Here's how the part is built. I have some questions about the finished solid (model axes, mm). Round coordinates to 2 decimals unless told otherwise and drop trailing zeros. Loops run counter-clockwise (first coordinate to the right, second up) from the corner with the lowest first, then second, coordinate; pieces in that order, holes last. Notation, with made-up numbers: (86.25, 73.5) - (101.25, 73.5) arc R17 cw to (101.25, 97.5) - close; hole circle Ø3 at (82, 83.25). An arc over 180 degrees is marked (long way). Answer as a JSON object with one key per item and string values. Group by question number.
1) I want a section at C-C, the plane y = -53.5. Please give me the cut outline in (x, z), then the cut area to 3 significant figures.
2) I want a section at A-A, the plane z = 255. Please give me the cut outline in (x, y).
3) I want a section at D-D, the plane z = 167. Please give me the cut outline in (x, y), then the cut area to 3 significant figures.
4) I want a section at B-B, the plane x = 0.1. Please give me the cut outline in (y, z).
5) Will these pins go through, and if not, where does the flat tip stop? P1, Ø1.5, axis at x = -1, z = 190.5, coming from the -Y side (3 decimals); P2, Ø0.9, axis at x = 0, z = 214.5, coming from the -Y side (3 decimals); P3, Ø0.9, axis at x = -0.5, y = 0, coming from the +Z side.
6) If I drill on line 1 along Y through (x, z) = (-1, 279.5); line 2 along Y through (x, z) = (0.5, 181); line 3 along Z through (x, y) = (0.15, -130), over which ranges is the centre line in solid material (lowest first)? Write a range as [from, to].
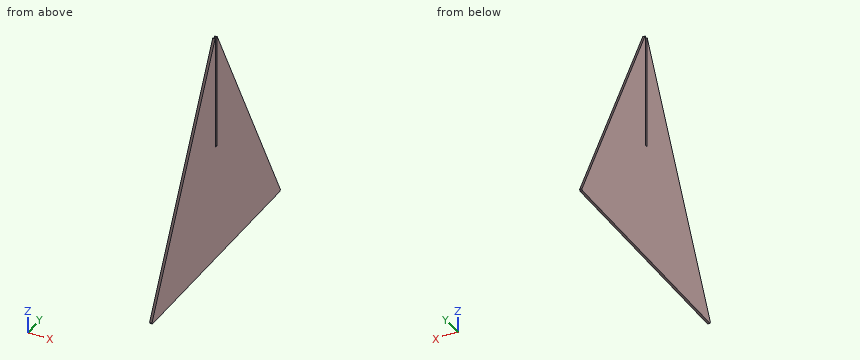
Autodesk Inventor part; units mm, degrees
ref_plane "YZ Plane" through (0, 0, 0) normal (1, 0, 0) x (0, 1, 0)
ref_plane "XZ Plane" through (0, 0, 0) normal (0, 1, 0) x (-1, 0, 0)
ref_plane "XY Plane" through (0, 0, 0) normal (0, 0, 1) x (1, 0, 0)
sketch "Sketch1" plane through (0, 0, 0) normal (1, 0, 0) x (0, 1, 0)
  line L0 (150, 0) -> (-150, 0)
  line L1 (0, 0) -> (0, 300)
  line L2 (0, 300) -> (150, 0)
  line L3 (0, 300) -> (-150, 0)
  dimension "d0" = 300
  dimension "d1" = 300
extrude "Plate1" add sketch "Sketch1" along normal mid plane 3
sketch "Sketch2" plane through (-1.5, 0, 0) normal (-1, 0, 0) x (0, 0, 1)
  line L0 (300, -1.6) -> (149, -1.6)
  line L1 (149, -1.6) -> (149, 1.6)
  line L2 (149, 1.6) -> (300, 1.6)
  line L3 (300, 1.6) -> (300, -1.6)
  point P0 (0, 0)
  point P1 (300, 0)
  point P2 (300, 0)
  dimension "d3" = 3.2
  dimension "d4" = 151
extrude "Extrusion1" cut sketch "Sketch2" against normal through all
chamfer "Corner Chamfer1" distance 2 angle 45 4 edges at (0, -1.6, 296.8) (0, 1.6, 296.8) (0, 150, 0) (0, -150, 0)
equation "\"d2\" = Thickness"
equation "\"BendReliefWidth\" = Thickness"
equation "\"BendReliefDepth\" = 0.5 * Thickness"
equation "\"CornerReliefSize\" = 4 * Thickness"
equation "\"MinimumRemnant\" = 2 * Thickness"
equation "\"TransitionRadius\" = BendRadius"
equation "\"JacobiRadiusSize\" = BendRadius"
equation "\"GapSize\" = Thickness"
properties part number "MSC 205 CONE BLADE" material "Stainless Steel"
Outcome:
{
 "1": {"outline": "(-1.5, 0) - (1.5, 0) - (1.5, 193) - (-1.5, 193) - close", "area": "579 mm^2"},
 "2": {"outline": "(-1.5, -22.5) - (1.5, -22.5) - (1.5, -1.6) - (-1.5, -1.6) - close; (-1.5, 1.6) - (1.5, 1.6) - (1.5, 22.5) - (-1.5, 22.5) - close"},
 "3": {"outline": "(-1.5, -66.5) - (1.5, -66.5) - (1.5, -1.6) - (-1.5, -1.6) - close; (-1.5, 1.6) - (1.5, 1.6) - (1.5, 66.5) - (-1.5, 66.5) - close", "area": "389 mm^2"},
 "4": {"outline": "(-149.11, 1.79) - (-148, 0) - (148, 0) - (149.11, 1.79) - (2.49, 295.01) - (1.6, 294.8) - (1.6, 149) - (-1.6, 149) - (-1.6, 294.8) - (-2.49, 295.01) - close"},
 "5": {"P1": "y = -55.125", "P2": "y = -42.975", "P3": "z = 149"},
 "6": {"line 1": "[-10.25, -1.6], [1.6, 10.25]", "line 2": "[-59.5, -1.6], [1.6, 59.5]", "line 3": "[0, 40]"}
}
